Source: CAD feature listing. Evaluate the final solid. Frame: model axes, mm. A direction names the side the tool comes from. Round coordinates to 2 decimals unless told otherwise and drop trailing zeros. Write each loop counter-clockwise with the first axis right and the second up, starting at its lowest first coordinate (ties: lowest second). Pieces come first, ordered by that corner, then holes. Notation, with made-up numbers: (41, -5) - (87, -5) arc R12 cw to (87, 7) - close; hole circle Ø2 at (18, 53.5). An arc over 180 degrees is marked (long way). Write item = value, one per line. Start each with the question number.
```python
from build123d import *

# Parameters (mm, degrees)
F0_W     = 16
F0_H     = 5
F1_DEPTH = 25.5
F2_W     = 45.2
F2_H     = 42.82105
F3_DEPTH = 34.2
F4_R     = 2.5
F5_DEPTH = 2.001
F6_R     = 5


with BuildPart() as f1:
    # F0 (on Right) → F1 (new body, symmetric)
    with BuildSketch(Plane.YZ):
        with BuildLine():
            Line((-14, 34.369719), (-14, 0))
            Line((-14, 0), (14, 0))
            Line((14, 0), (14, 34.369719))
            ThreePointArc((14, 34.369719), (13.463923, 35.663923), (12.169719, 36.2))
            Line((12.169719, 36.2), (5, 36.2))
            ThreePointArc((5, 36.2), (0, 31.2), (-5, 36.2))
            Line((-5, 36.2), (-12.169719, 36.2))
            ThreePointArc((-12.169719, 36.2), (-13.463923, 35.663923), (-14, 34.369719))
        make_face()
        with Locations((0, 15.5)):
            Rectangle(F0_W, F0_H, mode=Mode.SUBTRACT)
        with Locations((0, 25.5)):
            Rectangle(F0_W, F0_H, mode=Mode.SUBTRACT)
    extrude(amount=F1_DEPTH, both=True)

    # F2 (on face) → F3 (cut)
    with BuildSketch(Plane.XY.offset(36.2)):
        with Locations((0, 0.389209)):
            Rectangle(F2_W, F2_H)
    extrude(amount=-F3_DEPTH, mode=Mode.SUBTRACT)

    # F4 (on face) → F5 (cut, through all)
    with BuildSketch(Plane.XY.offset(2)):
        Circle(F4_R)
    extrude(amount=-F5_DEPTH, mode=Mode.SUBTRACT)

    # F6
    f6_edges = [f1.edges().sort_by_distance(p)[0] for p in [
        (25.5, 0, 0),
        (22.6, 0, 2),
        (-22.6, 0, 2),
        (-25.5, 0, 0),
    ]]
    fillet(f6_edges, radius=F6_R)


solid = f1.part
```
(1) Section D-D (y = 10.25). Return the cut outline in (x, z), plus the area to 3 significant figures.
(2) Reachability of faces 1 (the cylindrical face through (24.07, 0.2, 1.5)), 2 (the cylindrical face through (-21.17, 0.2, 3.5)), 3 (the flat face through (24, 8, 25)) from +Z, -Z, +X, -X, +Y, -Y: full face, straight path, thin tool, end or side. Return the list, or none.
(3) Pull-direction query (Y, two-part tool) for faces 4 (the flat face through (24, 0, 28)), 5 (the cylindrical face through (-24, 0.1, 31.2)), 6 (the cylindrical face through (24, -13, 36)), 7 (the cylindrical face through (24, 13, 36)); classes: +Y half, -Y half, draft (parallel to the pull), parting line (faces both ways), or undercut.
(4) Contact query for flat-ended pins moving along their axis: P1, Ø1.4, axis at x = 24, y = -3, coming from the +Z side; P2, Ø0.9, axis at x = 24.5, y = -1.5, coming from the -Z side; P3, Ø6, axis at x = 0, y = 0, coming from the +Z side. Output: stop coordinate, or through.
(5) Section B-B (z = 27). Return the cut outline in (x, y), plus the area to 3 significant figures.
(6) Section A-A (y = 0). Count the separate pieces of the cut face and the enclosed holes in it, plus the area to 3 significant figures.
(7) Ray query, L1, parallel to Y at x = 0, z = 1.35; L2, parallel to X at y = -11.75, z = 15.5; L3, parallel to Z at x = 9.5, y = 8. Return the intervals inside material, ascending. Write a range as from..to.
(8) Section C-C (x = 0). Return the cut outline in (y, z).
Solution:
q1.outline = (-25.5, 5) arc R5 ccw to (-20.5, 0) - (20.5, 0) arc R5 ccw to (25.5, 5) - (25.5, 36.2) - (22.6, 36.2) - (22.6, 7) arc R5 cw to (17.6, 2) - (-17.6, 2) arc R5 cw to (-22.6, 7) - (-22.6, 36.2) - (-25.5, 36.2) - close
q1.area = 300 mm^2
q2.face_1 = -Z, +X, +Y, -Y
q2.face_2 = +Z, +Y, -Y
q2.face_3 = +X, -X
q3.face_4 = undercut
q3.face_5 = undercut
q3.face_6 = -Y half
q3.face_7 = +Y half
q4.P1 = 32.84
q4.P2 = 1.48
q4.P3 = 2
q5.outline = (-25.5, -14) - (-22.6, -14) - (-22.6, -8) - (-25.5, -8) - close; (-25.5, 8) - (-22.6, 8) - (-22.6, 14) - (-25.5, 14) - close; (22.6, -14) - (25.5, -14) - (25.5, -8) - (22.6, -8) - close; (22.6, 8) - (25.5, 8) - (25.5, 14) - (22.6, 14) - close
q5.area = 69.6 mm^2
q6.separate_pieces = 6
q6.enclosed_holes = 0
q6.area = 203 mm^2
q7.L1 = -14..-2.5, 2.5..14
q7.L2 = -25.5..-22.6, 22.6..25.5
q7.L3 = 0..2
q8.outline = (-14, 0) - (-2.5, 0) - (-2.5, 2) - (-14, 2) - close; (2.5, 0) - (14, 0) - (14, 2) - (2.5, 2) - close
